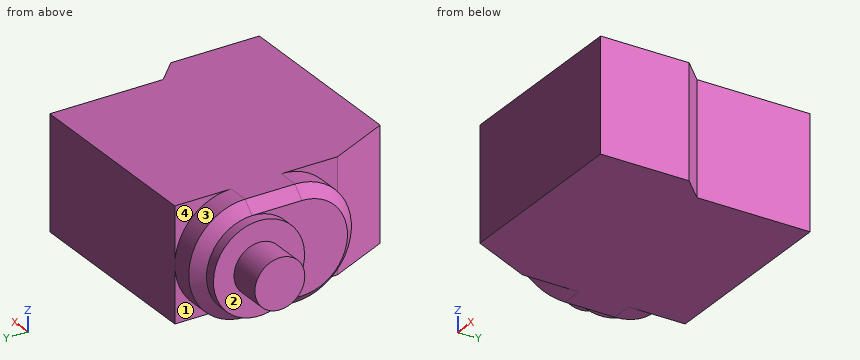
Autodesk Inventor part; units mm, degrees
ref_plane "YZ Plane" through (0, 0, 0) normal (1, 0, 0) x (0, 1, 0)
ref_plane "XZ Plane" through (0, 0, 0) normal (0, 1, 0) x (-1, 0, 0)
ref_plane "XY Plane" through (0, 0, 0) normal (0, 0, 1) x (1, 0, 0)
sketch "Sketch1" plane through (0, 0, 0) normal (0, 0, 1) x (1, 0, 0)
  line L0 (-8.128, -13.081) -> (11.43, -13.081)
  line L1 (11.43, -0.182) -> (11.43, 13.081)
  line L2 (11.43, 13.081) -> (-11.43, 13.081)
  line L3 (-11.43, 13.081) -> (-11.43, -5.969)
  line L4 (11.43, -13.081) -> (-8.128, -13.081)
  line L5 (-8.128, -13.081) -> (-11.43, -5.969)
  line L6 (11.43, -13.081) -> (13.97, -13.081)
  line L7 (13.97, -13.081) -> (13.97, -2.722)
  line L8 (13.97, -2.722) -> (11.43, -0.182)
  point P0 (0, 0)
  point P1 (0, -13.081)
  point P2 (-11.43, 0)
  dimension "d0" = 22.86
  dimension "d1" = 26.162
  dimension "d2" = 19.558
  dimension "d3" = 7.112
  dimension "d4" = 135
  dimension "d5" = 2.54
extrude "Extrusion1" add sketch "Sketch1" along normal mid plane 13.208
sketch "Sketch2" plane through (-11.43, -5.969, -6.604) normal (-1, 0, 0) x (0, 0, 1)
  line L0 (13.208, 0) -> (13.208, 19.05)
  line L1 (0, 19.05) -> (13.208, 19.05)
  line L2 (0, 19.05) -> (0, 0)
  line L3 (0, 0) -> (13.208, 0)
  arc A0 (0, 6.604) -> (13.208, 6.604) centre (6.604, 6.604) ccw
  arc A1 (13.208, 12.446) -> (0, 12.446) centre (6.604, 12.446) ccw
  point P0 (6.604, 5.969)
extrude "Extrusion2" add sketch "Sketch2" along normal blind 3.81 contours A0 L2 A1 L0
chamfer "Chamfer1" distance 1.27 angle 45 4 edges at (-15.24, 13.081, 0) (-15.24, 3.556, 6.604) (-15.24, -5.969, 0) (-15.24, 3.556, -6.604)
sketch "Sketch4" plane through (-15.24, -5.969, -6.604) normal (-1, 0, 0) x (0, 0, 1)
  arc A0 (11.938, 12.446) -> (1.27, 12.446) centre (6.604, 12.446) ccw
  circle A1 centre (6.604, 12.446) radius 5.334
  point P0 (6.604, 5.969)
extrude "Extrusion3" add sketch "Sketch4" along normal blind 1.27
sketch "Sketch5" plane through (-16.51, 6.477, 0) normal (-1, 0, 0) x (0, 0, 1)
  circle A0 centre (0, 0) radius 5.334
  circle A1 centre (0, 0) radius 2.921
  point P0 (0, -6.477)
  dimension "d15" = 5.842
extrude "Extrusion4" add sketch "Sketch5" along normal blind 3.81 contours A1
properties part number "Servo"
Part model, mm, in its own coordinate system. Face numbers are marked on the shaded views. A direction names the side the tool comes from. Give positions to 0.01 mm unless a question says otherwise; leave off trailing zeros. Loops run counter-clockwise (first coordinate to the right, second up) from the corner with the lowest first, then second, coordinate; pieces in that order, holes last. Notation, with made-up numbers: M 69.5,44.5 L 93.5,44.5 A20 ccw 93.5,77.5 Z; hole C 86.25,53.25 d9. An arc over 180 degrees is marked long. Return JSON: item names as keys, results as strings.
1) Saw through at A-A, the plane x = -9.5. List the corners of the cut face in (y, z).
Calculated:
{"outline": "M -10.13,-6.6 L 13.08,-6.6 L 13.08,6.6 L -10.13,6.6 Z"}
2) Flat gauge pins, fed straight in: pin 1 Ø5 at (y, z) = (7, -0.5) entering from +X; pin 2 Ø3.5 at (y, z) = (-1.5, -4) entering from -X. Where does each tip first touch, or does it go through?
Calculated:
{"pin 1": "stops at x = 11.43", "pin 2": "stops at x = -15.24"}
3) 3-axis set-ups, long thin cutter, end or side, ignore diameter. For the marked faces 1, 2, 3 and 4: which of +Z, -Z, +X, -X, +Y, -Y reach the whole face in a straight line?
Calculated:
{"face 1": "-Z, -X, +Y", "face 2": "-X", "face 3": "-X, +Y", "face 4": "+Z, -X, +Y"}
4) Drill centre lines: line 1 (X direction, y = -3, z = -3.75); line 2 (X direction, y = 11, z = -2.5); line 3 (Y direction, x = -14, z = 5). Where is each one in solid material? Low to high.
Calculated:
{"line 1": "x = -15.24 to 13.97", "line 2": "x = -16.51 to 11.43", "line 3": "y = -3.63 to 10.75"}
